Part model, mm, in its own coordinate system. Face numbers are marked on the shaded views. A direction names the side the tool comes from. Round coordinates to 2 decimals unless told otherwise and drop trailing zeros. Loops run counter-clockwise (first coordinate to the right, second up) from the corner with the lowest first, then second, coordinate; pieces in that order, holes last.
1) Drop flat-ended pins along their axis: P1, Ø2, axis at y = 2, z = 2.5, coming from the -X side; P2, Ø1, axis at x = 0.5, y = 17, coming from the +Z side; P3, Ø6.5, axis at x = 0.5, y = 16.5, coming from the -Z side. Give the stop position or say it passes through.
2) Band-saw the part on C-C, the plane y = 7.5. Write the cut outline in (x, z), then the cut area to 3 significant figures.
3) 3-axis set-ups, long thin cutter, end or side, ignore diameter. For the marked faces 5, 6 and 7: which of +Z, -Z, +X, -X, +Y, -Y reach the whole face in a straight line?
4) Probe line 1 (X direction, y = 2.75, z = 0); line 2 (Y direction, x = 3.5, z = 2); line 3 (Z direction, x = -0.5, y = 9.5). List the from-to ranges inside material, lowest first.
5) Band-saw the part on D-D, the plane y = 11.75. Write the cut outline in (x, z), then the cut area to 3 significant figures.
6) Band-saw the part on B-B, the plane x = 0. Write the cut outline in (y, z), then the cut area to 3 significant figures.
7) Band-saw the part on A-A, the plane z = 0. Write the cut outline in (x, y).
8) Mould opens along Z. For the marked faces 1, 2, 3 and 4 say: +Z half, -Z half, draft (parallel to the pull), parting line (faces both ways), or undercut.
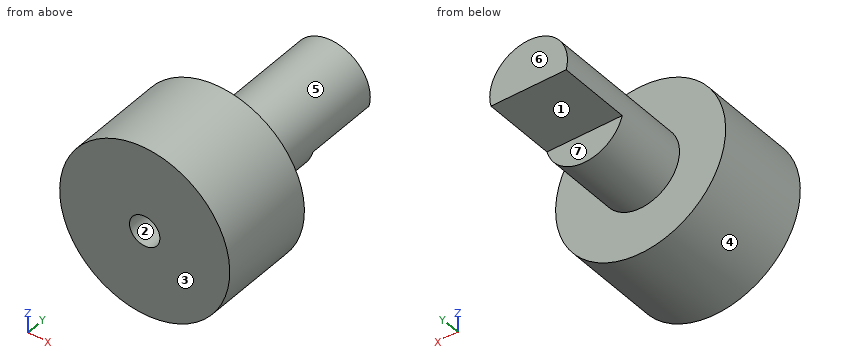
from build123d import *

# Parameters (mm, degrees)
SKETCH1_R           = 7
BOSS_EXTRUDE1_DEPTH = 8
SKETCH2_R           = 3.2
BOSS_EXTRUDE2_DEPTH = 12
SKETCH3_W           = 6.196773354
SKETCH3_H           = 3.205100748
CUT_EXTRUDE1_DEPTH  = 6
SKETCH4_R           = 1.25
CUT_EXTRUDE2_DEPTH  = 10


with BuildPart() as part:
    # Sketch1 → Boss-Extrude1 (new body)
    with BuildSketch(Plane(origin=(0, 0, 0), x_dir=(1, 0, 0), z_dir=(0, 1, 0))):
        with Locations(Location((0, 0, 0), (0, 0, 270))):
            Circle(SKETCH1_R)
    extrude(amount=BOSS_EXTRUDE1_DEPTH)

    # Sketch2 → Boss-Extrude2 (add)
    with BuildSketch(Plane(origin=(0, 8, 0), x_dir=(1, 0, 0), z_dir=(0, 1, 0))):
        with Locations(Location((0, 0, 0), (0, 0, 270))):
            Circle(SKETCH2_R)
    extrude(amount=BOSS_EXTRUDE2_DEPTH)

    # Sketch3 → Cut-Extrude1 (cut)
    with BuildSketch(Plane(origin=(0, 20, 0), x_dir=(1, 0, 0), z_dir=(0, 1, 0))):
        with Locations((0, 2.402550374)):
            Rectangle(SKETCH3_W, SKETCH3_H)
    extrude(amount=-CUT_EXTRUDE1_DEPTH, mode=Mode.SUBTRACT)

    # Sketch4 → Cut-Extrude2 (cut)
    with BuildSketch(Plane.XZ):
        with Locations(Location((0, 0, 0), (0, 0, 270))):
            Circle(SKETCH4_R)
    extrude(amount=-CUT_EXTRUDE2_DEPTH, mode=Mode.SUBTRACT)


solid = part.part
Reported:
1. P1: stops at x = -6.84
1. P2: stops at z = 3.2
1. P3: stops at z = -3.2
2. outline: circle Ø14 at (0, 0); hole circle Ø2.5 at (0, 0)
2. area: 149 mm2
3. face 5: +Y
3. face 6: +Z, -Z, +X, -X, +Y
3. face 7: -Z, +X, -X, +Y
4. line 1: x = -7 to -1.25, 1.25 to 7
4. line 2: y = 0 to 8
4. line 3: z = -3.16 to -1.15, 1.15 to 3.16
5. outline: circle Ø6.4 at (0, 0)
5. area: 32.2 mm2
6. outline: (0, -7) - (8, -7) - (8, -3.2) - (14, -3.2) - (14, -0.8) - (20, -0.8) - (20, 3.2) - (8, 3.2) - (8, 7) - (0, 7) - (0, 1.25) - (10, 1.25) - (10, -1.25) - (0, -1.25) - close
6. area: 149 mm2
7. outline: (-7, 0) - (-1.25, 0) - (-1.25, 10) - (1.25, 10) - (1.25, 0) - (7, 0) - (7, 8) - (3.2, 8) - (3.2, 20) - (-3.2, 20) - (-3.2, 8) - (-7, 8) - close
8. face 1: -Z half
8. face 2: undercut
8. face 3: draft
8. face 4: parting line
